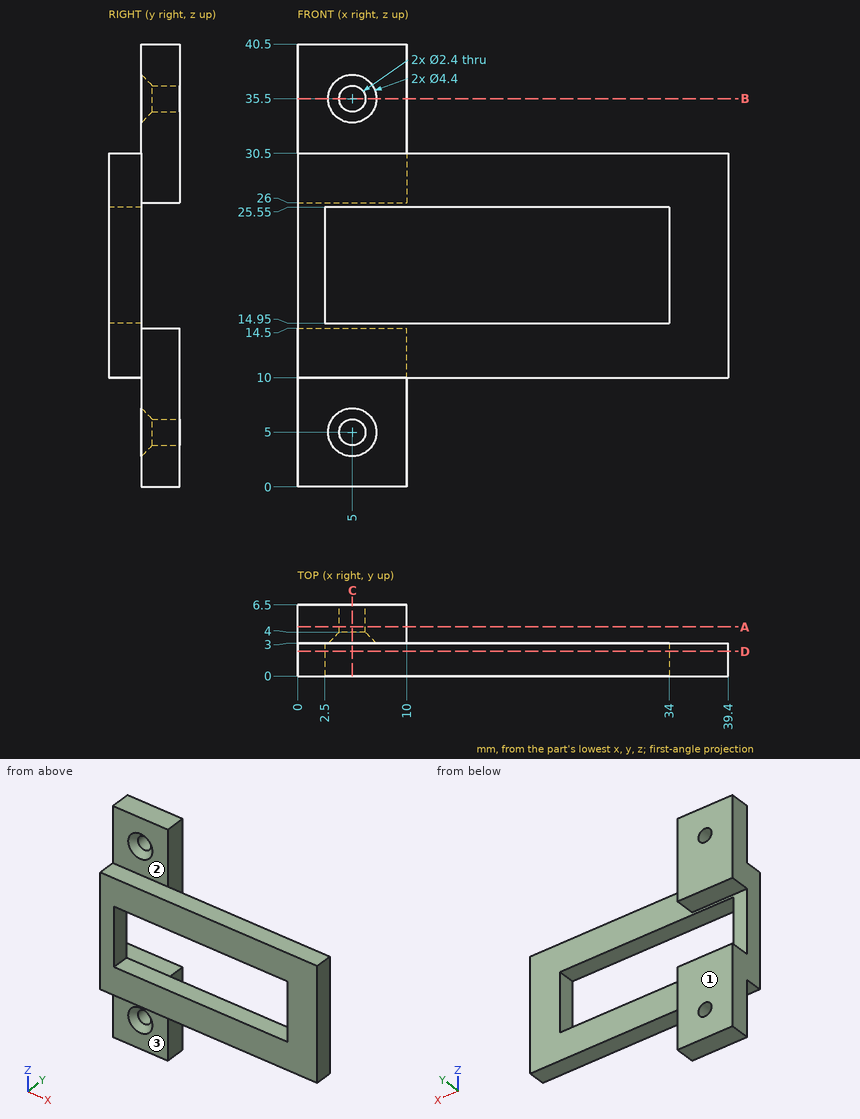
Verification items for this drawing (mm, ordinates from the low corner). A direction names the side the tool comes from. Coordinates: 2 decimals unless noted, no trailing zeros. Order: outer loops, then holes, each group sorted by start corner. A loop starts at its lowest first (then second) coordinate and runs counter-clockwise, first axis right, second up. Notation, with made-up numbers: (73.25, -25.5) - (92.25, -25.5) arc R16 ccw to (92.25, -7.5) - close; hole circle Ø10 at (-19.5, 14.25). An arc over 180 degrees is marked (long way). Answer in a Markdown table with one row per item. Add a question column.
1. Access from +Z, -Z, +X, -X, +Y, -Y to the whole of each face (thin tool, end or side, straight path). Record for the marked faces 1, 2 and 3.
2. Gauge pin test, flat ends, axial feed: pin 1 Ø3 at (x, z) = (4.5, 25) entering from -Y; pin 2 Ø3.5 at (x, y) = (25, 2) entering from -Z; pin 3 Ø1 at (y, z) = (4, 5) entering from +X; pin 4 Ø2.5 at (x, y) = (19, 1.5) entering from +Z. Record the tip position at first contact, or that the pin passes through.
3. Section check C-C (x = 5). Enter the section's corners in (y, z).
4. Material ranges on L1, parallel to Z at x = 5, y = 4.85; L2, parallel to Z at x = 17.5, y = 2.5; L3, parallel to X at y = 5.5, z = 5, recorded low to high. Write a range as [from, to].
5. Section check D-D (y = 2.25). Enter the section's corners in (x, z).
6. Section check B-B (z = 35.5). Enter the section's corners in (x, y).
7. Section check A-A (y = 4.5). Enter the section's corners in (x, z), plus the area to 3 significant figures.
Data:
| question | item | result |
|---|---|---|
| 1 | face 1 | +Z, -Z, +X, -X, +Y |
| 1 | face 2 | +Z, +X, -X, -Y |
| 1 | face 3 | -Z, +X, -X, -Y |
| 2 | pin 1 | stops at y = 0 |
| 2 | pin 2 | stops at z = 10 |
| 2 | pin 3 | stops at x = 10 |
| 2 | pin 4 | stops at z = 30.5 |
| 3 | outline | (0, 10) - (3, 10) - (3, 7.2) - (4, 6.2) - (6.5, 6.2) - (6.5, 14.5) - (3, 14.5) - (3, 14.95) - (0, 14.95) - close; (0, 25.55) - (3, 25.55) - (3, 26) - (6.5, 26) - (6.5, 34.3) - (4, 34.3) - (3, 33.3) - (3, 30.5) - (0, 30.5) - close; (3, 0) - (6.5, 0) - (6.5, 3.8) - (4, 3.8) - (3, 2.8) - close; (3, 37.7) - (4, 36.7) - (6.5, 36.7) - (6.5, 40.5) - (3, 40.5) - close |
| 4 | L1 | z = [0, 3.8], [6.2, 14.5], [26, 34.3], [36.7, 40.5] |
| 4 | L2 | z = [10, 14.95], [25.55, 30.5] |
| 4 | L3 | x = [0, 3.8], [6.2, 10] |
| 5 | outline | (0, 10) - (39.4, 10) - (39.4, 30.5) - (0, 30.5) - close; hole (2.5, 14.95) - (34, 14.95) - (34, 25.55) - (2.5, 25.55) - close |
| 6 | outline | (0, 3) - (2.8, 3) - (3.8, 4) - (3.8, 6.5) - (0, 6.5) - close; (6.2, 4) - (7.2, 3) - (10, 3) - (10, 6.5) - (6.2, 6.5) - close |
| 7 | outline | (0, 0) - (10, 0) - (10, 14.5) - (0, 14.5) - close; (0, 26) - (10, 26) - (10, 40.5) - (0, 40.5) - close; hole circle Ø2.4 at (5, 5); hole circle Ø2.4 at (5, 35.5) |
| 7 | area | 281 mm² |
